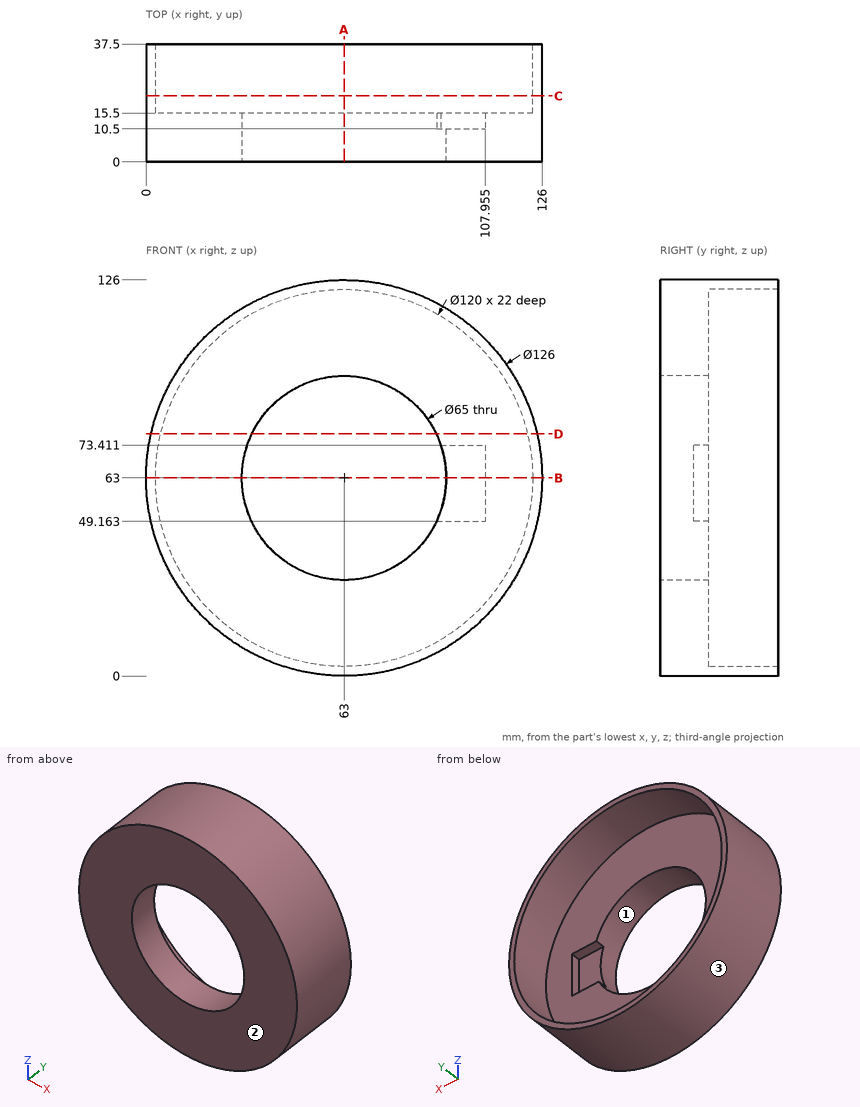
Could you check a few things on this drawing? It's one solid part, dimensions in mm from its lowest x, y, z. Round coordinates to 2 decimals unless told otherwise and drop trailing zeros. Loops run counter-clockwise (first coordinate to the right, second up) from the corner with the lowest first, then second, coordinate; pieces in that order, holes last. Notation, with made-up numbers: (71.5, 77.25) -> (88.5, 77.25) arc R27 ccw to (88.5, 116.25) -> close; hole circle Ø10 at (51, -33). An arc over 180 degrees is marked (long way). One line per item, written item: value. Start each with the question number.
1. If I drill on probe 1 along X at (y, z) = (21, 63); probe 2 along Z at (x, y) = (63, 8.5), over which ranges is the centre line in solid material (lowest first)?
2. If we section it at B-B, the plane z = 63: Write out the boundary of the cut face in (x, y) (1 decimal), then the cut area to 3 significant figures.
3. If we mould it in two halves opening along X, with no side actions, what happens to the marked faces 1, 2 and 3? For each: pulls with the +X half, pulls with the -X half, needs draft (parallel to the pull), parting line crosses it, or undercut.
4. For pin 1 (2 mm diameter, centred on x = 32, y = 17, fed in from -Z); pin 2 (17 mm diameter, centred on x = 97, z = 55.5, fed in from +Y); pin 3 (4 mm diameter, centred on x = 101.5, y = 12.5, fed in from -Z), each with a flat end and sliding along its axis, tell me the tip position at first contact or that it passes through.
5. If we section it at D-D, the plane z = 77: Write out the boundary of the cut face in (x, y) (1 decimal).
6. If we section it at A-A, the plane x = 63: Write out the boundary of the cut face in (y, z).
7. If we section it at C-C, the plane y = 21: Write out the boundary of the cut face in (x, z), then the cut area to 3 significant figures.
Calculated:
1. probe 1: x = 0 to 3, 123 to 126
1. probe 2: z = 0 to 30.5, 95.5 to 126
2. outline: (0, 0) -> (30.5, 0) -> (30.5, 15.5) -> (3, 15.5) -> (3, 37.5) -> (0, 37.5) -> close; (95.5, 0) -> (126, 0) -> (126, 37.5) -> (123, 37.5) -> (123, 15.5) -> (108, 15.5) -> (108, 10.5) -> (95.5, 10.5) -> close
2. area: 1,020 mm²
3. face 1: undercut
3. face 2: needs draft
3. face 3: parting line crosses it
4. pin 1: stops at z = 7.6
4. pin 2: stops at y = 15.5
4. pin 3: stops at z = 11.65
5. outline: (1.6, 0) -> (33.7, 0) -> (33.7, 15.5) -> (4.7, 15.5) -> (4.7, 37.5) -> (1.6, 37.5) -> close; (92.3, 0) -> (124.4, 0) -> (124.4, 37.5) -> (121.3, 37.5) -> (121.3, 15.5) -> (92.3, 15.5) -> close
6. outline: (0, 0) -> (37.5, 0) -> (37.5, 3) -> (15.5, 3) -> (15.5, 30.5) -> (0, 30.5) -> close; (0, 95.5) -> (15.5, 95.5) -> (15.5, 123) -> (37.5, 123) -> (37.5, 126) -> (0, 126) -> close
7. outline: circle Ø126 at (63, 63); hole circle Ø120 at (63, 63)
7. area: 1,160 mm²
